```python
from build123d import *

# Parameters (mm, degrees)
CROQUIS1_W              = 152.4
CROQUIS1_H              = 114.3
SALIENTE_EXTRUIR1_DEPTH = 12.7
CROQUIS3_R              = 10.16
CORTAR_EXTRUIR1_DEPTH   = 97.092936785
SALIENTE_EXTRUIR2_DEPTH = 50.8
CORTAR_EXTRUIR2_DEPTH   = 148.45007773


with BuildPart() as part:
    # Croquis1 → Saliente-Extruir1 (new body)
    with BuildSketch(Plane(origin=(0, 0, 0), x_dir=(1, 0, 0), z_dir=(0, 1, 0))):
        Rectangle(CROQUIS1_W, CROQUIS1_H)
    extrude(amount=SALIENTE_EXTRUIR1_DEPTH)

    # Croquis3 → Cortar-Extruir1 (cut, through all)
    with BuildSketch(Plane(origin=(0, 12.7, 0), x_dir=(1, 0, 0), z_dir=(0, 1, 0))):
        with Locations(Location((50.8, -31.75, 0), (0, 0, 270))):
            Circle(CROQUIS3_R)
        with BuildLine():
            Line((-76.2, -21.59), (-50.8, -21.59))
            ThreePointArc((-50.8, -21.59), (-40.64, -31.75), (-50.8, -41.91))
            Line((-50.8, -41.91), (-76.2, -41.91))
            Line((-76.2, -41.91), (-76.2, -21.59))
        make_face()
    cortar_extruir1 = extrude(amount=-CORTAR_EXTRUIR1_DEPTH, mode=Mode.SUBTRACT)

    # Simetría1: Cortar-Extruir1 across plane
    add(cortar_extruir1.mirror(Plane.XY), mode=Mode.SUBTRACT)

    # Croquis4 → Saliente-Extruir2 (add)
    with BuildSketch(Plane(origin=(0, 12.7, 0), x_dir=(1, 0, 0), z_dir=(0, 1, 0))):
        Polygon((53.881536726, 0), (0, -53.881536726), (-53.881536726, 0), (0, 53.881536726), align=None)
    extrude(amount=SALIENTE_EXTRUIR2_DEPTH)

    # Croquis5 → Cortar-Extruir2 (cut, through all)
    with BuildSketch(Plane(origin=(26.940768363, 0, 26.940768363), x_dir=(0.7071067811865464, 0, -0.7071067811865488), z_dir=(0.7071067811865488, 0, 0.7071067811865464))):
        Polygon((-31.75, 63.5), (31.75, 63.5), (3.175, 34.925), (3.175, 29.21), (-3.175, 29.21), (-3.175, 34.925), align=None)
    extrude(amount=-CORTAR_EXTRUIR2_DEPTH, mode=Mode.SUBTRACT)


solid = part.part
```
Here's how the part is built. I have some questions about the finished solid (model axes, mm). A direction names the side the tool comes from. Coordinates: 2 decimals unless noted, no trailing zeros. Order: outer loops, then holes, each group sorted by start corner. A loop starts at its lowest first (then second) coordinate and runs counter-clockwise, first axis right, second up.
1) Imagine slicing it at C-C on z = -9. List the corners of the cut face in (x, y) for me (3 decimals), and give its area (3 significant figures).
2) Will these pins go through, and if not, where does the flat tip stop? pin 1 (1 mm diameter, centred on x = 21.5, z = -7, fed in from +Y); pin 2 (4 mm diameter, centred on x = -41.5, z = -4.5, fed in from +Y); pin 3 (1.5 mm diameter, centred on y = 20.5, z = -26, fed in from +X); pin 4 (16.5 mm diameter, centred on x = 50.8, z = 31.75, fed in from +Y).
3) Imagine slicing it at B-B on z = -31.75. List the corners of the cut face in (x, y) for me, and give its area (3 significant figures).
4) I need wall thicknesses on line 1 (Z direction, x = 50, y = 4); line 2 (X direction, y = 4, z = -31); line 3 (X direction, y = 4.5, z = 31.75). Which ranges of each line are inside material? Lowest first, please.
5) Imagine slicing it at D-D on x = -10. List the corners of the cut face in (y, z) for me (3 decimals), and give its area (3 significant figures).
6) Imagine slicing it at A-A on x = -58. List the corners of the cut face in (y, z) for me, and give its area (3 significant figures).
7) Which directions (+Z, -Z, +X, -X, +Y, -Y) give clear straight access to the entire face, cutting with the end or side of a thin tool? Please do faces 4 (the face through (2.62, 32.11, -1.87)), 5 (the face through (-27.32, 26.46, -26.56)), 6 (the face through (27.32, 26.46, 26.56)), 7 (the face through (-64, 6, -21.59)).
8) We'd pull the mould along X, two halves only. Please class faces 1 (the face through (-76.2, 6, -49)), 2 (the face through (-1, 0, -1)), 3 (the face through (-1.87, 32.03, 2.62)): +X half, -X half, draft (parallel to the pull), parting line (faces both ways), or undercut.
Response values:
1. outline: (-76.2, 0) - (76.2, 0) - (76.2, 12.7) - (44.882, 12.7) - (44.882, 63.5) - (35.901, 63.5) - (-4.51, 34.925) - (-4.51, 29.21) - (-13.49, 29.21) - (-13.49, 34.925) - (-44.882, 57.122) - (-44.882, 12.7) - (-76.2, 12.7) - close
1. area: 5,060 mm2
2. pin 1: stops at y = 52.4
2. pin 2: stops at y = 59.91
2. pin 3: stops at x = 28.63
2. pin 4: passes through
3. outline: (-40.64, 0) - (40.64, 0) - (40.64, 12.7) - (22.13, 12.7) - (22.13, 63.5) - (13.15, 63.5) - (-22.13, 38.55) - (-22.13, 12.7) - (-40.64, 12.7) - close; (60.96, 0) - (76.2, 0) - (76.2, 12.7) - (60.96, 12.7) - close
3. area: 3,030 mm2
4. line 1: z = -57.15 to -41.88, -21.62 to 21.62, 41.88 to 57.15
4. line 2: x = -40.67 to 40.67, 60.93 to 76.2
4. line 3: x = -40.64 to 40.64, 60.96 to 76.2
5. outline: (0, -57.15) - (12.7, -57.15) - (12.7, -43.882) - (55.708, -43.882) - (34.925, -14.49) - (29.21, -14.49) - (29.21, -5.51) - (34.925, -5.51) - (63.5, 34.901) - (63.5, 43.882) - (12.7, 43.882) - (12.7, 57.15) - (0, 57.15) - close
5. area: 4,490 mm2
6. outline: (0, -57.15) - (12.7, -57.15) - (12.7, -41.91) - (0, -41.91) - close; (0, -21.59) - (12.7, -21.59) - (12.7, 21.59) - (0, 21.59) - close; (0, 41.91) - (12.7, 41.91) - (12.7, 57.15) - (0, 57.15) - close
6. area: 935 mm2
7. face 4: +Y
7. face 5: -Z, -X, +Y
7. face 6: +Z, +X, +Y
7. face 7: -X, +Y, -Y
8. face 1: -X half
8. face 2: draft
8. face 3: undercut
